For this review, use the dimensioned drawing (mm, ordinates from the lowest corner) and the shaded views. A direction names the side the tool comes from. Coordinates: 2 decimals unless noted, no trailing zeros. Write each loop counter-clockwise with the first axis right and the second up, starting at its lowest first coordinate (ties: lowest second). Pieces come first, ordered by that corner, then holes. Notation, with made-up numbers: M 23.5,-10 L 75.5,-10 A34 cw 75.5,28 Z; hole C 42.25,69 d1. An arc over 180 degrees is marked long. Return JSON: item names as keys, results as strings. Group by question number.
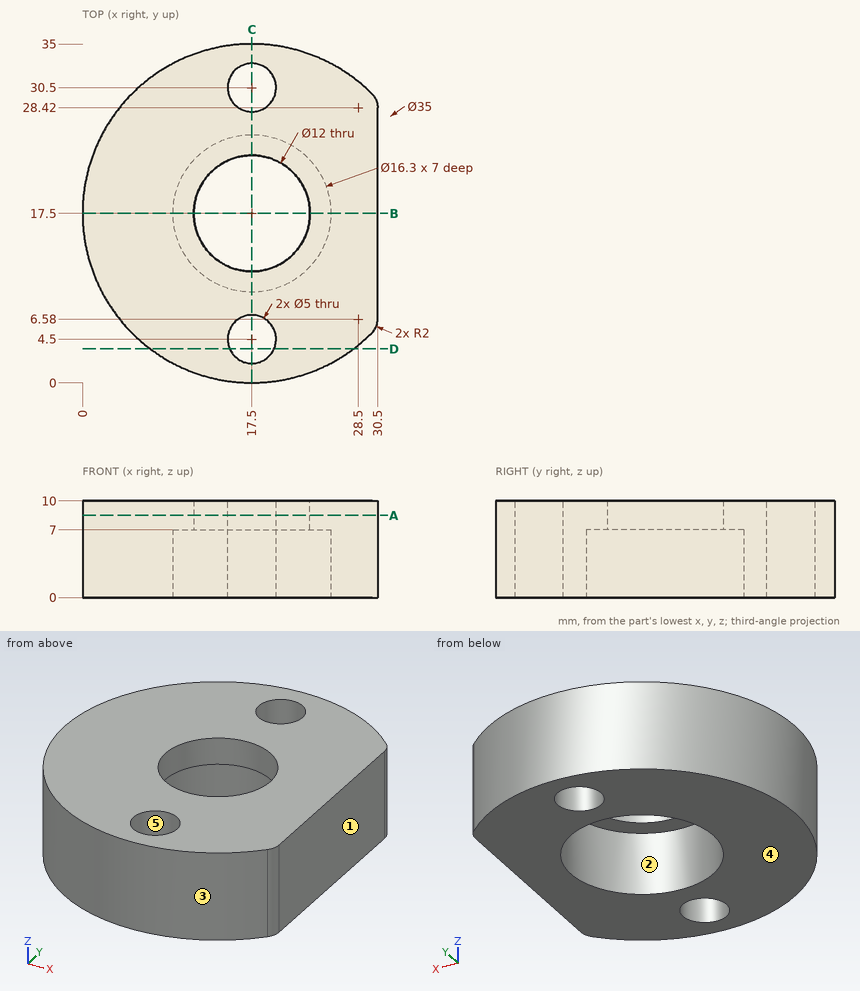
Item 1: For pin 1 (8 mm diameter, centred on x = 20, y = 18, fed in from -Z); pin 2 (5 mm diameter, centred on y = 6.5, z = 8, fed in from -X); pin 3 (4 mm diameter, centred on x = 7, z = 9, fed in from -Y), all flat-tipped, find the tip position at first contact; note any pin that passes through.
Item 2: Machinability: for the marked faces 1 and 2, which of the approach directions +Z, -Z, +X, -X, +Y, -Y give a long, thin tool a straight path to every point of the face, cutting with its end or side? Answer none if there is none.
Item 3: The part is to be moulded in two halves that separate along Y. For the marked faces 3, 4 and 5, say which applies: pulls with the +Y half, pulls with the -Y half, needs draft (parallel to the pull), parting line crosses it, or undercut.
Item 4: For line 1 (Y direction, x = 17.5, z = 5.25); line 2 (Y direction, x = 15.5, z = 1.25) (1 decimal); line 3 (X direction, y = 30.5, z = 7.5) (1 decimal), list the stretches that pass through material, from the lowest coordinate up.
Item 5: Add section A-A (z = 8.5). Write out the cut boundary in (x, y), plus the area to 3 significant figures.
Item 6: Add section D-D (y = 3.5). Write out the cut boundary in (x, z).
Item 7: Add section B-B (y = 17.5). Write out the cut boundary in (x, z), plus the area to 3 significant figures.
Item 8: Add section C-C (x = 17.5). Write out the cut boundary in (y, z), plus the area to 3 significant figures.
Geometry check:
{
 "1": {"pin 1": "z = 7", "pin 2": "x = 2.2", "pin 3": "y = 2.2"},
 "2": {"face 1": "+Z, -Z, +X, +Y, -Y", "face 2": "-Z"},
 "3": {"face 3": "parting line crosses it", "face 4": "needs draft", "face 5": "undercut"},
 "4": {"line 1": "0 to 2, 7 to 9.35, 25.65 to 28, 33 to 35", "line 2": "0.1 to 3, 6 to 9.6, 25.4 to 29, 32 to 34.9", "line 3": "5.8 to 15, 20 to 29.2"},
 "5": {"outline": "M 29.92,5.17 A2 ccw 30.5,6.58 L 30.5,28.42 A2 ccw 29.92,29.83 A17.5 ccw long Z; hole C 17.5,17.5 d12; hole C 17.5,4.5 d5; hole C 17.5,30.5 d5", "area": "737 mm^2"},
 "6": {"outline": "M 7,0 L 15.21,0 L 15.21,10 L 7,10 Z; M 19.79,0 L 28,0 L 28,10 L 19.79,10 Z"},
 "7": {"outline": "M 0,0 L 9.35,0 L 9.35,7 L 11.5,7 L 11.5,10 L 0,10 Z; M 23.5,7 L 25.65,7 L 25.65,0 L 30.5,0 L 30.5,10 L 23.5,10 Z", "area": "155 mm^2"},
 "8": {"outline": "M 0,0 L 2,0 L 2,10 L 0,10 Z; M 7,0 L 9.35,0 L 9.35,7 L 11.5,7 L 11.5,10 L 7,10 Z; M 23.5,7 L 25.65,7 L 25.65,0 L 28,0 L 28,10 L 23.5,10 Z; M 33,0 L 35,0 L 35,10 L 33,10 Z", "area": "99.9 mm^2"}
}
